```python
from build123d import *

# Parameters (mm, degrees)
CIRPATTERN1_COUNT = 8
CIRPATTERN2_COUNT = 6


with BuildPart() as part:
    # Sketch1 → Revolve1 (revolve)
    with BuildSketch(Plane(origin=(0, 0, 0), x_dir=(0, 0, -1), z_dir=(1, 0, 0)), mode=Mode.PRIVATE) as revolve1_sk:
        Polygon((0, 32), (0, 44), (-5, 44), (-5, 41), (-1.5, 41), (-1.5, 38), (-1, 38), (-1, 32), align=None)
    revolve(revolve1_sk.sketch.rotate(Axis((0, 0, 0), (0, 0, 1)), 90), axis=Axis((0, 0, 0), (0, 0, 1)))

    # Sketch2 → Ø3.0 (3) Diameter Hole1 (revolve, cut)
    with BuildSketch(Plane(origin=(0, 35, 1), x_dir=(0, -1, 0), z_dir=(1, 0, 0))):
        Polygon((0, 0), (0, 2.401290929), (1.5, 1.5), (1.5, 0), align=None)
    f_3_0_3_diameter_hole1 = revolve(axis=Axis((0, 35, 7.35), (0, 0, -1)), mode=Mode.SUBTRACT)

    # CirPattern1: Ø3.0 (3) Diameter Hole1 ×8 about axis
    cirpattern1_axis = Axis((0, 0, 0), (0, 0, 1))
    for i in range(1, CIRPATTERN1_COUNT):
        add(f_3_0_3_diameter_hole1.rotate(cirpattern1_axis, i * 360 / CIRPATTERN1_COUNT), mode=Mode.SUBTRACT)

    # Sketch4 → M2.5x0.45 Tapped Hole1 (revolve, cut)
    with BuildSketch(Plane(origin=(0, 44, 3), x_dir=(0, 0, 1), z_dir=(1, 0, 0))):
        Polygon((0, 0), (0, 6.965882135), (1.025, 6.35), (1.025, 0), align=None)
    m2_5x0_45_tapped_hole1 = revolve(axis=Axis((0, 50.35, 3), (0, -1, 0)), mode=Mode.SUBTRACT)

    # CirPattern2: M2.5x0.45 Tapped Hole1 ×6 about axis
    cirpattern2_axis = Axis((0, 0, 5.25), (0, 0, -1))
    for i in range(1, CIRPATTERN2_COUNT):
        add(m2_5x0_45_tapped_hole1.rotate(cirpattern2_axis, i * 360 / CIRPATTERN2_COUNT), mode=Mode.SUBTRACT)


solid = part.part
```
The model under review builds one solid part; all positions refer to its coordinate system, in mm. A direction names the side the tool comes from. Round coordinates to 2 decimals unless told otherwise and drop trailing zeros. Write each loop counter-clockwise with the first axis right and the second up, starting at its lowest first coordinate (ties: lowest second). Pieces come first, ordered by that corner, then holes.
(1) We need section A-A on x = 0. Give the number of separate pieces and of enclosed holes in the cut face, and give its area (3 significant figures).
(2) We need section B-B on y = 0. Give the boundary of the cut face in (x, z).
(3) We need section C-C on z = 3. Give the boundary of the cut face in (x, y) (3 decimals), and give its area (3 significant figures).
(4) Mouldability with a two-part tool opening along Z and no side actions: class faces 3 (the flat face through (36, -20, 5)), 4 (the cylindrical face through (-36.2, 0.9, 0.5)), 5 (the cylindrical face through (37.25, -20.51, 3.55)) as +Z half, -Z half, draft (parallel to the pull), parting line (faces both ways), or undercut.
(5) Insertion check: pin 1 (2.5 mm diameter, centred on x = 0, y = 35, fed in from +Z); pin 2 (3.5 mm diameter, centred on x = -24.75, y = -24.75, fed in from -Z); pin 3 (3.5 mm diameter, centred on x = 24.75, y = 24.75, fed in from +Z); pin 4 (1 mm diameter, centred on y = 14, z = 3.5, fed in from +X). Each pin has a flat end and moves straight along its axis. Give the tip position at first contact, or say it passes through.
(6) Machinability: for faces 1 (the flat face through (-12, 36.3, 1.5)), 2 (the flat face through (-23, 23, 0)), which of the approach directions +Z, -Z, +X, -X, +Y, -Y give a long, thin tool a straight path to every point of the face, cutting with its end or side? Answer none if there is none.
(7) We need section D-D on y = -13.5. Give the boundary of the cut face in (x, z).
(8) Wall thickness on L1, parallel to Y at x = 0, z = 0.2; L2, parallel to Z at x = 0, y = 42.6 (3 decimals); L3, parallel to X at y = 1, z = 4.8: over which ranges is each line inside the solid? List them lowest first.
Findings below:
1. separate pieces: 6
1. enclosed holes: 0
1. area: 32.7 mm2
2. outline: (-44, 0) - (-36.5, 0) - (-36.5, 1) - (-38, 1) - (-38, 1.5) - (-41, 1.5) - (-41, 5) - (-44, 5) - close; (-33.5, 0) - (-32, 0) - (-32, 1) - (-33.5, 1) - close; (32, 0) - (33.5, 0) - (33.5, 1) - (32, 1) - close; (36.5, 0) - (44, 0) - (44, 5) - (41, 5) - (41, 1.5) - (38, 1.5) - (38, 1) - (36.5, 1) - close
3. outline: (-38.607, -21.106) - (-36.008, -19.606) arc R41 cw to (-36.008, 19.606) - (-38.607, 21.106) arc R44 ccw to start; (-37.582, -22.882) arc R44 ccw to (-1.025, -43.988) - (-1.025, -40.987) arc R41 cw to (-34.983, -21.381) - close; (-37.582, 22.882) - (-34.983, 21.381) arc R41 cw to (-1.025, 40.987) - (-1.025, 43.988) arc R44 ccw to start; (1.025, -43.988) arc R44 ccw to (37.582, -22.882) - (34.983, -21.381) arc R41 cw to (1.025, -40.987) - close; (1.025, 40.987) arc R41 cw to (34.983, 21.381) - (37.582, 22.882) arc R44 ccw to (1.025, 43.988) - close; (36.008, -19.606) - (38.607, -21.106) arc R44 ccw to (38.607, 21.106) - (36.008, 19.606) arc R41 cw to start
3. area: 764 mm2
4. face 3: +Z half
4. face 4: draft
4. face 5: undercut
5. pin 1: passes through
5. pin 2: stops at z = 0
5. pin 3: stops at z = 1
5. pin 4: stops at x = 41.88
6. face 1: +Z
6. face 2: -Z, +X, -X, +Y, -Y
7. outline: (-41.88, 0) - (-29.01, 0) - (-29.01, 1) - (-35.52, 1) - (-35.52, 1.5) - (-38.71, 1.5) - (-38.71, 5) - (-41.88, 5) - close; (29.01, 0) - (41.88, 0) - (41.88, 5) - (38.71, 5) - (38.71, 1.5) - (35.52, 1.5) - (35.52, 1) - (29.01, 1) - close
8. L1: y = -44 to -36.5, -33.5 to -32, 32 to 33.5, 36.5 to 44
8. L2: z = 0 to 1.975, 4.025 to 5
8. L3: x = -43.99 to -40.99, 40.99 to 43.99
